The model under review builds one solid part; all positions refer to its coordinate system, in mm. A direction names the side the tool comes from. Give positions to 0.01 mm unless a question says otherwise; leave off trailing zeros. Loops run counter-clockwise (first coordinate to the right, second up) from the corner with the lowest first, then second, coordinate; pieces in that order, holes last. Notation, with made-up numbers: (67.25, 84) -> (111.25, 84) arc R21 cw to (111.25, 97) -> close; hole circle Ø11 at (-13, -16). An arc over 180 degrees is marked (long way). Write each question's results on one line, items separated by ' | '. Start each with the question number.
Q1. We need section C-C (z = 6.5). Write out the cut boundary in (x, y).
Q2. We need section B-B (x = 57). Write out the cut boundary in (y, z), plus the area to 3 significant figures.
Q3. Insertion check: pin 1 Ø5 at (x, z) = (-49.5, 5) entering from -Y; pin 2 Ø9 at (x, y) = (-10, 9) entering from +Z; pin 3 Ø1.5 at (y, z) = (19, -8.5) entering from +X. Each pin has a flat end and moves straight along its axis. Give the tip position at first contact, or say it passes through.
Q4. We need section A-A (y = 10.5). Write out the cut boundary in (x, z), plus the area to 3 significant figures.
Q5. Wall thickness on L1, parallel to Z at x = -59, y = 6; L2, parallel to Y at x = -94, z = 11.25; L3, parallel to X at y = 9, z = -9.75: over which ranges is each line inside the solid? List them lowest first. Write a range as [from, to].
Q6. Machinability: for faces 1 (the face through (140, 18, 1)), 2 (the face through (2, 18, 7)), which of the approach directions +Z, -Z, +X, -X, +Y, -Y give a long, thin tool a straight path to every point of the face, cutting with its end or side? Answer none if there is none.
from build123d import *

# Parameters (mm, degrees)
SKETCH1_W           = 280
SKETCH1_H           = 25
BOSS_EXTRUDE1_DEPTH = 30
SKETCH2_W           = 10.5
SKETCH2_H           = 18
CUT_EXTRUDE1_DEPTH  = 300
CHAMFER1_SIZE       = 6.5


with BuildPart() as part:
    # Sketch1 → Boss-Extrude1 (new body)
    with BuildSketch(Plane(origin=(0, 0, 0), x_dir=(1, 0, 0), z_dir=(0, 1, 0))):
        Rectangle(SKETCH1_W, SKETCH1_H)
    extrude(amount=BOSS_EXTRUDE1_DEPTH)

    # Sketch2 → Cut-Extrude1 (cut)
    with BuildSketch(Plane(origin=(140, 0, 0), x_dir=(0, 0, -1), z_dir=(1, 0, 0))):
        with Locations((-7.25, 9)):
            Rectangle(SKETCH2_W, SKETCH2_H)
    extrude(amount=-CUT_EXTRUDE1_DEPTH, mode=Mode.SUBTRACT)

    # Chamfer1
    chamfer1_edges = [part.edges().sort_by_distance(p)[0] for p in [
        (-140, 15, -12.5),
        (140, 15, -12.5),
    ]]
    chamfer(chamfer1_edges, length=CHAMFER1_SIZE)


solid = part.part
Output:
1) outline: (-140, 18) -> (140, 18) -> (140, 30) -> (-140, 30) -> close
2) outline: (0, -12.5) -> (30, -12.5) -> (30, 12.5) -> (18, 12.5) -> (18, 2) -> (0, 2) -> close | area: 561 mm2
3) pin 1: y = 18 | pin 2: z = 2 | pin 3: x = 138.25
4) outline: (-140, -6) -> (-133.5, -12.5) -> (133.5, -12.5) -> (140, -6) -> (140, 2) -> (-140, 2) -> close | area: 4,020 mm2
5) L1: [-12.5, 2] | L2: [18, 30] | L3: [-136.25, 136.25]
6) face 1: +Z, -Z, +X, +Y, -Y | face 2: +Z, +X, -X, -Y
